Verification items for the finished model (mm, model axes). Face numbers are marked on the shaded views. Round coordinates to 2 decimals unless told otherwise and drop trailing zeros. Order: outer loops, then holes, each group sorted by start corner. A loop starts at its lowest first (then second) coordinate and runs counter-clockwise, first axis right, second up. Notation, with made-up numbers: (3.5, -25) -> (21.5, -25) arc R16 cw to (21.5, -15) -> close; hole circle Ø6 at (-35.75, -37). An arc over 180 degrees is marked (long way). Put each result on its own line as item: value.
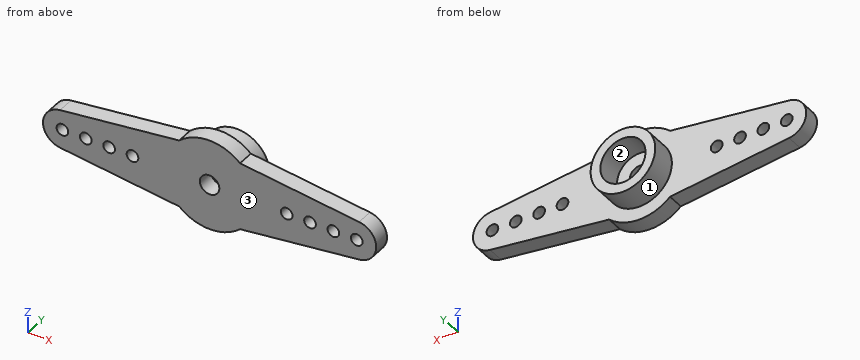
```python
from build123d import *

# Parameters (mm, degrees)
SKETCH1_R           = 5.85
SKETCH1_R_2         = 1.25
SKETCH1_R_3         = 0.75
BOSS_EXTRUDE1_DEPTH = 2.15
SKETCH2_R           = 4.15
SKETCH2_R_2         = 2.9
BOSS_EXTRUDE2_DEPTH = 3.3


with BuildPart() as part:
    # Sketch1 → Boss-Extrude1 (new body)
    # profile 1 of 3: a face of its own
    with BuildSketch(Plane(origin=(0, 0, 0), x_dir=(1, 0, 0), z_dir=(0, 1, 0))):
        Circle(SKETCH1_R)
        with Locations(Location((0, 0, 0), (0, 0, 90))):
            Circle(SKETCH1_R_2, mode=Mode.SUBTRACT)
    # profile 2 of 3: a face of its own
    with BuildSketch(Plane(origin=(0, 0, 0), x_dir=(1, 0, 0), z_dir=(0, 1, 0))):
        with BuildLine():
            Line((-3.911521443, 4.35), (-19.203214028, 2.481544127))
            ThreePointArc((-19.203214028, 2.481544127), (-21.4, 0), (-19.203214028, -2.481544127))
            Line((-19.203214028, -2.481544127), (-3.911521443, -4.35))
            ThreePointArc((-3.911521443, -4.35), (-5.85, 0), (-3.911521443, 4.35))
        make_face()
        with Locations(Location((-18.9, 0, 0), (0, 0, 90))):
            Circle(SKETCH1_R_3, mode=Mode.SUBTRACT)
        with Locations(Location((-15.9, 0, 0), (0, 0, 90))):
            Circle(SKETCH1_R_3, mode=Mode.SUBTRACT)
        with Locations(Location((-12.9, 0, 0), (0, 0, 90))):
            Circle(SKETCH1_R_3, mode=Mode.SUBTRACT)
        with Locations(Location((-9.9, 0, 0), (0, 0, 90))):
            Circle(SKETCH1_R_3, mode=Mode.SUBTRACT)
    # profile 3 of 3: a face of its own
    with BuildSketch(Plane(origin=(0, 0, 0), x_dir=(1, 0, 0), z_dir=(0, 1, 0))):
        with BuildLine():
            Line((19.203214028, 2.481544127), (3.911521443, 4.35))
            ThreePointArc((3.911521443, 4.35), (5.343449281, 2.381186633), (5.85, 0))
            ThreePointArc((5.85, 0), (5.343449281, -2.381186633), (3.911521443, -4.35))
            Line((3.911521443, -4.35), (19.203214028, -2.481544127))
            ThreePointArc((19.203214028, -2.481544127), (21.4, 0), (19.203214028, 2.481544127))
        make_face()
        with Locations(Location((9.9, 0, 0), (0, 0, 90))):
            Circle(SKETCH1_R_3, mode=Mode.SUBTRACT)
        with Locations(Location((12.9, 0, 0), (0, 0, 90))):
            Circle(SKETCH1_R_3, mode=Mode.SUBTRACT)
        with Locations(Location((15.9, 0, 0), (0, 0, 90))):
            Circle(SKETCH1_R_3, mode=Mode.SUBTRACT)
        with Locations(Location((18.9, 0, 0), (0, 0, 90))):
            Circle(SKETCH1_R_3, mode=Mode.SUBTRACT)
    extrude(amount=BOSS_EXTRUDE1_DEPTH)

    # Sketch2 → Boss-Extrude2 (add)
    with BuildSketch(Plane(origin=(0, 2.15, 0), x_dir=(1, 0, 0), z_dir=(0, 1, 0))):
        with Locations(Location((0, 0, 0), (0, 0, 270))):
            Circle(SKETCH2_R)
        with Locations(Location((0, 0, 0), (0, 0, 270))):
            Circle(SKETCH2_R_2, mode=Mode.SUBTRACT)
    extrude(amount=BOSS_EXTRUDE2_DEPTH)


solid = part.part
```
Item 1: Sectioned sample at C-C, the plane y = 3.85. Record the boundary of the cut face in (x, z), then the cut area to 3 significant figures.
Geometry check:
outline: circle Ø8.3 at (0, 0); hole circle Ø5.8 at (0, 0)
area: 27.7 mm2
Item 2: Sectioned sample at B-B, the plane z = 3.5. Record the boundary of the cut face in (x, y).
Geometry check:
outline: (-10.87, 0) -> (10.87, 0) -> (10.87, 2.15) -> (2.23, 2.15) -> (2.23, 5.45) -> (-2.23, 5.45) -> (-2.23, 2.15) -> (-10.87, 2.15) -> close
Item 3: Material ranges on line 1 along X through (y, z) = (4.4, 0); line 2 along Y through (x, z) = (10, 2.75); line 3 along Z through (x, y) = (-15.9, 0.6), recorded low to high.
Geometry check:
line 1: -4.15 to -2.9, 2.9 to 4.15
line 2: 0 to 2.15
line 3: -2.89 to -0.75, 0.75 to 2.89
Item 4: Release check for a two-part mould opening along Z. For the marked faces 1, 2 and 3 record: pulls with the +Z half, pulls with the -Z half, needs draft (parallel to the pull), parting line crosses it, or undercut.
Geometry check:
face 1: parting line crosses it
face 2: undercut
face 3: needs draft
Item 5: Depth check by flat-ended pin: pin 1 Ø3 at (x, z) = (0, 0) entering from +Y; pin 2 Ø1.5 at (y, z) = (4.5, 4.5) entering from +X; pin 3 Ø1 at (y, z) = (2.5, -0.5) entering from +X. Enter the tip coordinate at first touch or a pass-through.
Geometry check:
pin 1: y = 2.15
pin 2: x = 1.78
pin 3: x = 21.4
Item 6: Sectioned sample at D-D, the plane x = -12.9. Record the boundary of the cut face in (y, z).
Geometry check:
outline: (0, -3.25) -> (2.15, -3.25) -> (2.15, -0.75) -> (0, -0.75) -> close; (0, 0.75) -> (2.15, 0.75) -> (2.15, 3.25) -> (0, 3.25) -> close
Item 7: Sectioned sample at A-A, the plane x = 0. Record the boundary of the cut face in (y, z).
Geometry check:
outline: (0, -5.85) -> (2.15, -5.85) -> (2.15, -4.15) -> (5.45, -4.15) -> (5.45, -2.9) -> (2.15, -2.9) -> (2.15, -1.25) -> (0, -1.25) -> close; (0, 1.25) -> (2.15, 1.25) -> (2.15, 2.9) -> (5.45, 2.9) -> (5.45, 4.15) -> (2.15, 4.15) -> (2.15, 5.85) -> (0, 5.85) -> close
